from build123d import *

# Parameters (mm, degrees)
BOSS_EXTRUDE2_START = 5
SKETCH2_R           = 2.5
BOSS_EXTRUDE2_DEPTH = 5
FILLET1_R           = 5


with BuildPart() as part:
    # Sketch3 → Revolve1 (revolve)
    with BuildSketch(Plane.XY, mode=Mode.PRIVATE) as revolve1_sk:
        Polygon((0, 0), (-34, 0), (-34, 10), (-27.5, 16), (-27.5, 35), (0, 35), align=None)
    revolve(revolve1_sk.sketch.rotate(Axis((0, 67.276563105, 0), (0, -1, 0)), 270), axis=Axis((0, 67.276563105, 0), (0, -1, 0)))

    # Sketch2 → Boss-Extrude2 (add)
    with BuildSketch(Plane(origin=(0, 35, 0), x_dir=(1, 0, 0), z_dir=(0, 1, 0)).offset(BOSS_EXTRUDE2_START)):
        with BuildLine():
            ThreePointArc((31.556090162, 12.657534265), (34.641016151, 20), (26.739791304, 20.999608592))
            ThreePointArc((26.739791304, 20.999608592), (17, 29.444863729), (4.816298858, 33.657142857))
            ThreePointArc((4.816298858, 33.657142857), (0, 40), (-4.816298858, 33.657142857))
            ThreePointArc((-4.816298858, 33.657142857), (-17, 29.444863729), (-26.739791304, 20.999608592))
            ThreePointArc((-26.739791304, 20.999608592), (-34.641016151, 20), (-31.556090162, 12.657534265))
            ThreePointArc((-31.556090162, 12.657534265), (-34, 0), (-31.556090162, -12.657534265))
            ThreePointArc((-31.556090162, -12.657534265), (-34.641016151, -20), (-26.739791304, -20.999608592))
            ThreePointArc((-26.739791304, -20.999608592), (-17, -29.444863729), (-4.816298858, -33.657142857))
            ThreePointArc((-4.816298858, -33.657142857), (0, -40), (4.816298858, -33.657142857))
            ThreePointArc((4.816298858, -33.657142857), (17, -29.444863729), (26.739791304, -20.999608592))
            ThreePointArc((26.739791304, -20.999608592), (34.641016151, -20), (31.556090162, -12.657534265))
            ThreePointArc((31.556090162, -12.657534265), (34, 0), (31.556090162, 12.657534265))
        make_face()
        with Locations(Location((-30.310889132, -17.5, 0), (0, 0, 270))):
            Circle(SKETCH2_R, mode=Mode.SUBTRACT)
        with Locations(Location((-30.310889132, 17.5, 0), (0, 0, 270))):
            Circle(SKETCH2_R, mode=Mode.SUBTRACT)
        with Locations(Location((0, -35, 0), (0, 0, 270))):
            Circle(SKETCH2_R, mode=Mode.SUBTRACT)
        with Locations(Location((0, 35, 0), (0, 0, 270))):
            Circle(SKETCH2_R, mode=Mode.SUBTRACT)
        with Locations(Location((30.310889132, -17.5, 0), (0, 0, 270))):
            Circle(SKETCH2_R, mode=Mode.SUBTRACT)
        with Locations(Location((30.310889132, 17.5, 0), (0, 0, 270))):
            Circle(SKETCH2_R, mode=Mode.SUBTRACT)
    extrude(amount=-BOSS_EXTRUDE2_DEPTH)

    # Fillet1
    fillet1_edges = [part.edges().sort_by_distance(p)[0] for p in [
        (-4.816298858, 37.5, 33.657142857),
        (4.816298858, 37.5, 33.657142857),
        (26.739791304, 37.5, 20.999608592),
        (31.556090162, 37.5, 12.657534265),
        (31.556090162, 37.5, -12.657534265),
        (26.739791304, 37.5, -20.999608592),
        (4.816298858, 37.5, -33.657142857),
        (-4.816298858, 37.5, -33.657142857),
        (-26.739791304, 37.5, -20.999608592),
        (-31.556090162, 37.5, -12.657534265),
        (-31.556090162, 37.5, 12.657534265),
        (-26.739791304, 37.5, 20.999608592),
    ]]
    fillet(fillet1_edges, radius=FILLET1_R)


solid = part.part
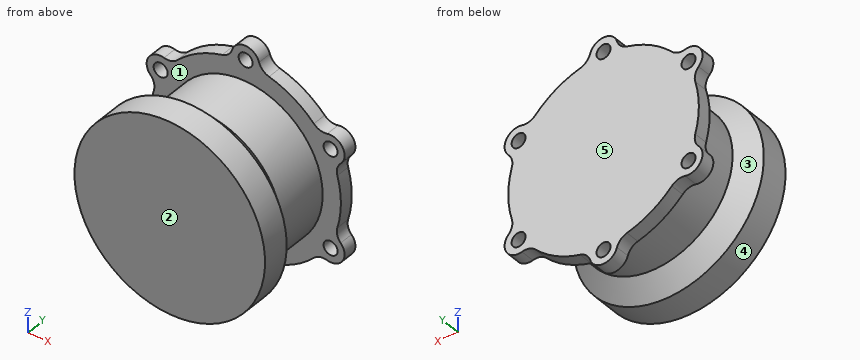
Geometry: final body of the model. Coordinates: model frame, mm. Face numbers are marked on the shaded views. A direction names the side the tool comes from. Round coordinates to 2 decimals unless told otherwise and drop trailing zeros. Order: outer loops, then holes, each group sorted by start corner. A loop starts at its lowest first (then second) coordinate and runs counter-clockwise, first axis right, second up. Notation, with made-up numbers: (75.5, 49.5) -> (86.5, 49.5) arc R30 cw to (86.5, 76.5) -> close; hole circle Ø1 at (79.5, -35). An arc over 180 degrees is marked (long way). Put each result on its own line as item: value. Start each with the question number.
Q1. Section A-A on x = 0. Return the cut outline in (y, z).
Q2. Line query: probe 1 along X at (y, z) = (36, -17); probe 2 along Y at (x, z) = (-30, -6.5); probe 3 along Y at (x, z) = (31.5, -9). Output: solid intervals per line, ascending.
Q3. Section B-B on y = 20.5. Return the cut outline in (x, z), and give its area (3 significant figures).
Q4. Section C-C on z = -17.5. Give the number of separate pieces and of enclosed holes in the cut face, and give its area (3 significant figures).
Q5. First-contact query: pin 1 (6 mm diameter, centred on x = 0, z = 35, fed in from -Y); pin 2 (3 mm diameter, centred on x = -30.31, z = 17.5, fed in from +Y); pin 3 (6 mm diameter, centred on y = 9.5, z = 4.5, fed in from -X); pin 4 (1.5 mm diameter, centred on x = 17, y = 26.5, fed in from +Z). Flat tips, straight axial feed; report the tip coordinate or a pass-through.
Q6. Pull-direction query (Y, two-part tool) for the marked faces 3, 4 and 5; classes: +Y half, -Y half, draft (parallel to the pull), parting line (faces both ways), or undercut.
Q7. Reachability of the marked faces 1 and 2 from +Z, -Z, +X, -X, +Y, -Y: full face, straight path, thin tool, end or side. Return the list, or none.
Ans:
1. outline: (0, -34) -> (10, -34) -> (16, -27.5) -> (35, -27.5) -> (35, -32.5) -> (40, -32.5) -> (40, 32.5) -> (35, 32.5) -> (35, 27.5) -> (16, 27.5) -> (10, 34) -> (0, 34) -> close; (35, -40) -> (40, -40) -> (40, -37.5) -> (35, -37.5) -> close; (35, 37.5) -> (40, 37.5) -> (40, 40) -> (35, 40) -> close
2. probe 1: x = -35.29 to -32.76, -27.86 to 27.86, 32.76 to 35.29
2. probe 2: y = 0 to 13.05, 35 to 40
2. probe 3: y = 0 to 11.14, 35 to 40
3. outline: circle Ø55 at (0, 0)
3. area: 2,380 mm2
4. separate pieces: 3
4. enclosed holes: 0
4. area: 2,000 mm2
5. pin 1: stops at y = 0
5. pin 2: stops at y = 10.46
5. pin 3: stops at x = -33.97
5. pin 4: stops at z = 22.19
6. face 3: undercut
6. face 4: draft
6. face 5: +Y half
7. face 1: none
7. face 2: +Z, -Z, +X, -X, -Y
